```python
from build123d import *

# Parameters (mm, degrees)
SALIENTE_EXTRUIR1_DEPTH = 2
SALIENTE_EXTRUIR2_DEPTH = 24
CROQUIS4_W              = 26.838471133
CROQUIS4_H              = 17.040828642
CORTAR_EXTRUIR1_DEPTH   = 70.1
SALIENTE_EXTRUIR3_DEPTH = 2
SALIENTE_EXTRUIR4_DEPTH = 2
CROQUIS7_W              = 45.5
CROQUIS7_H              = 2
SALIENTE_EXTRUIR5_DEPTH = 8
SALIENTE_EXTRUIR6_DEPTH = 6
CROQUIS9_W              = 76.962380363
CROQUIS9_H              = 58.957858246
CORTAR_EXTRUIR2_DEPTH   = 28


with BuildPart() as part:
    # Croquis1 → Saliente-Extruir1 (new body)
    with BuildSketch(Plane.XY):
        Polygon((-48.939551095, 26.503456625), (-8.439551095, 26.503456625), (-4.439551095, 26.503456625), (-4.439551095, 1.503456625), (-8.439551095, 1.503456625), (-49.939551095, 1.503456625), (-49.939551095, 5.503456625), (-49.939551095, 26.503456625), align=None)
    extrude(amount=SALIENTE_EXTRUIR1_DEPTH)

    # Croquis3 → Saliente-Extruir2 (add)
    with BuildSketch(Plane.XY):
        Polygon((-48.939551095, 26.503456625), (-8.439551095, 26.503456625), (-4.439551095, 26.503456625), (-4.439551095, 1.503456625), (-49.939551095, 1.503456625), (-49.939551095, 26.503456625), align=None)
        Polygon((-10.439551095, 3.503456625), (-47.939551095, 3.503456625), (-47.939551095, 5.503456625), (-47.939551095, 24.503456625), (-10.439551095, 24.503456625), (-6.439551095, 24.503456625), (-6.439551095, 3.503456625), align=None, mode=Mode.SUBTRACT)
    extrude(amount=SALIENTE_EXTRUIR2_DEPTH)

    # Croquis4 → Cortar-Extruir1 (cut)
    with BuildSketch(Plane(origin=(0, 0, 0), x_dir=(0, 0, -1), z_dir=(1, 0, 0))):
        with Locations((-15.419235567, 13.92807924)):
            Rectangle(CROQUIS4_W, CROQUIS4_H)
    extrude(amount=-CORTAR_EXTRUIR1_DEPTH, mode=Mode.SUBTRACT)

    # Croquis5 → Saliente-Extruir3 (add)
    with BuildSketch(Plane(origin=(0, 26.503456625, 0), x_dir=(1, 0, 0), z_dir=(0, 1, 0))):
        Polygon((-49.939551095, -20.607192887), (-4.439551095, -20.607192887), (-4.439551095, -36.1), (-8.439551095, -36.1), (-48.939551095, -36.1), (-49.939551095, -36.1), align=None)
    extrude(amount=-SALIENTE_EXTRUIR3_DEPTH)

    # Croquis6 → Saliente-Extruir4 (add)
    with BuildSketch(Plane.XY.offset(36.1)):
        Polygon((-4.439551095, 24.503456625), (-49.939551095, 24.503456625), (-49.939551095, 33.503456625), (-48.939551095, 33.503456625), (-8.439551095, 33.503456625), (-4.439551095, 33.503456625), align=None)
    extrude(amount=-SALIENTE_EXTRUIR4_DEPTH)

    # Croquis7 → Saliente-Extruir5 (add)
    with BuildSketch(Plane.XY.offset(36.1)):
        with Locations((-27.189551095, 32.503456625)):
            Rectangle(CROQUIS7_W, CROQUIS7_H)
    extrude(amount=-SALIENTE_EXTRUIR5_DEPTH)

    # Croquis8 → Saliente-Extruir6 (add)
    with BuildSketch(Plane.XY.offset(36.1)):
        Polygon((-49.939551095, 29.503456625), (-49.939551095, 26.503456625), (-49.715027183, 26.503456625), (-8.439551095, 26.503456625), (-4.439551095, 26.503456625), (-4.439551095, 29.503456625), (-8.439551095, 29.503456625), (-49.715027183, 29.503456625), align=None)
    extrude(amount=-SALIENTE_EXTRUIR6_DEPTH)

    # Croquis9 → Cortar-Extruir2 (cut)
    with BuildSketch(Plane.XY.offset(24)):
        with Locations((-25.38769132, 23.863692023)):
            Rectangle(CROQUIS9_W, CROQUIS9_H)
    extrude(amount=CORTAR_EXTRUIR2_DEPTH, mode=Mode.SUBTRACT)


solid = part.part
```
Work out the finished part from the listing and answer in its coordinate system (mm). A direction names the side the tool comes from. Give positions to 0.01 mm unless a question says otherwise; leave off trailing zeros. Loops run counter-clockwise (first coordinate to the right, second up) from the corner with the lowest first, then second, coordinate; pieces in that order, holes last. Notation, with made-up numbers: (-27.5, -38) - (24.5, -38) arc R16 cw to (24.5, -33) - close; hole circle Ø9 at (34, 31). An arc over 180 degrees is marked (long way). Use CSV: the item, a comma, the result in double quotes. Start each with the question number.
(1) A tool of negligible diameter and unlimited length cuts with its end or side. For faces 1 (the face through (-6.44, 23, 13)), 2 (the face through (-49, 5.408, 13)), 3 (the face through (-27, 3, 24)), from which of +Z, -Z, +X, -X, +Y, -Y can it reach the whole face along a straight path? Write none if from no direction.
(2) Find section C-C, the plane y = 23. Determine the outline of the cut face in (x, z).
(3) Find section A-A, the plane z = 3.25. Determine the outline of the cut face in (x, y), plus the area to 3 significant figures.
(4) Determine the mould class of faces 4 (the face through (-28, 1.503, 12)), 5 (the face through (-4.44, 23, 9)), 6 (the face through (-47.94, 4, 13)) for opening direction Y: released by +Y, released by -Y, zero draft, split by the parting line, or undercut.
(5) Find section B-B, the plane x = -28. Determine the outline of the cut face in (y, z).
(6) Find section D-D, the plane y = 13.5. Determine the outline of the cut face in (x, z), plus the area to 3 significant figures.
(7) This flat-tipped pin is pushed along its axis until it touches: pin 1 (8 mm diameter, centred on x = -38.5, y = 17, fed in from +Z). Where does it stop, or does it pass through?
(8) Find the intervals of material crossed by L1, parallel to Y at x = -17, z = 21.75; L2, parallel to Z at x = -31, y = 22.25; L3, parallel to X at y = 4.75, z = 7, in increasing order.
Results found:
1,face 1,"+Z"
1,face 2,"+Z, +X, -X"
1,face 3,"+Z, +X, -X, +Y, -Y"
2,outline,"(-49.94, 0) - (-4.44, 0) - (-4.44, 24) - (-6.44, 24) - (-6.44, 2) - (-47.94, 2) - (-47.94, 24) - (-49.94, 24) - close"
3,outline,"(-49.94, 1.5) - (-4.44, 1.5) - (-4.44, 5.41) - (-6.44, 5.41) - (-6.44, 3.5) - (-47.94, 3.5) - (-47.94, 5.41) - (-49.94, 5.41) - close; (-49.94, 22.45) - (-47.94, 22.45) - (-47.94, 24.5) - (-6.44, 24.5) - (-6.44, 22.45) - (-4.44, 22.45) - (-4.44, 26.5) - (-49.94, 26.5) - close"
3,area,"198 mm^2"
4,face 4,"released by -Y"
4,face 5,"zero draft"
4,face 6,"undercut"
5,outline,"(1.5, 0) - (26.5, 0) - (26.5, 24) - (24.5, 24) - (24.5, 2) - (3.5, 2) - (3.5, 24) - (1.5, 24) - close"
6,outline,"(-49.94, 0) - (-4.44, 0) - (-4.44, 2) - (-49.94, 2) - close"
6,area,"91.0 mm^2"
7,pin 1,"z = 2"
8,L1,"1.5 to 3.5, 24.5 to 26.5"
8,L2,"0 to 2"
8,L3,"-49.94 to -47.94, -6.44 to -4.44"
